Work out the finished part from the listing and answer in its coordinate system (mm). Give positions to 0.01 mm unless a question says otherwise; leave off trailing zeros. Write each loop counter-clockwise with the first axis right and the second up, starting at its lowest first coordinate (ties: lowest second). Pieces come first, ordered by that corner, then holes. Notation, with made-up numbers: (37, 12) - (58, 12) arc R9 cw to (58, 24) - close; hole circle Ø7 at (-20, -17). An arc over 180 degrees is marked (long way). Write item = value, one per line.
from build123d import *


with BuildPart() as part:
    # Skica1 → Rotovat1 (revolve)
    with BuildSketch(Plane.XY, mode=Mode.PRIVATE) as rotovat1_sk:
        with BuildLine():
            Line((-14.349982858, 244.001851534), (-13.849982858, 271.001851534))
            ThreePointArc((-13.849982858, 271.001851534), (-13.849828576, 271.018515344), (-13.849982858, 271.035179154))
            Line((-13.849982858, 271.035179154), (-13.75, 271.037030688))
            ThreePointArc((-13.75, 271.037030688), (-13.749828576, 271.018515344), (-13.75, 271))
            Line((-13.75, 271), (-14.25, 244))
            ThreePointArc((-14.25, 244), (-14.620475493, 230.995018288), (-15.25, 218))
            Line((-15.25, 218), (-15.349829703, 218.005833564))
            ThreePointArc((-15.349829703, 218.005833564), (-14.72040161, 230.9988616), (-14.349982858, 244.001851534))
        make_face()
    revolve(rotovat1_sk.sketch.rotate(Axis((0, 0, 0), (0, 1, 0)), 270), axis=Axis((0, 0, 0), (0, 1, 0)))


solid = part.part
1. Find section B-B, the plane y = 256.5. Give the vertices of the cut face in (x, z).
Solution:
outline = circle Ø28.24 at (0, 0); hole circle Ø28.04 at (0, 0)
2. Find section A-A, the plane y = 236.5. Give the vertices of the cut face in (x, z), then the cut area to 3 significant figures.
Solution:
outline = circle Ø29.06 at (0, 0); hole circle Ø28.86 at (0, 0)
area = 9.10 mm^2
3. Given pin 1 (12 mm diameter, centred on y = 244, z = 8.5, fed in from -X); pin 2 (5 mm diameter, centred on x = -5.5, y = 254.5, fed in from -Z); pin 3 (1.5 mm diameter, centred on x = 0, y = 241, fed in from -Z), each flat-ended and moving along its own axis, determine where each tip first touches the part or whether it passes through.
Solution:
pin_1 = -14.14
pin_2 = -13.84
pin_3 = -14.43
4. Straight lines are drawn through the part: line 1 (X direction, y = 235, z = -11); line 2 (X direction, y = 268, z = -10.5); line 3 (Z direction, x = 11.5, y = 252.5). For each, find the intervals that lie inside material, in ascending order.
Solution:
line_1 = -9.57 to -9.41, 9.41 to 9.57
line_2 = -9.12 to -8.96, 8.96 to 9.12
line_3 = -8.32 to -8.15, 8.15 to 8.32
